from build123d import *

# Parameters (mm, degrees)
F1_DEPTH  = 8
F2_R      = 5.45
F3_DEPTH  = 1
F3_TAPER  = 20
F5_DEPTH  = 1
F5_TAPER  = 20
F6_R      = 2.15
F7_DEPTH  = 0.63
F8_W      = 90.39
F8_H      = 51.7
F9_DEPTH  = 1.5
F11_DEPTH = 0.58


with BuildPart() as f1:
    # F0 (on Front) → F1 (new body)
    with BuildSketch(Plane.XZ):
        with BuildLine():
            ThreePointArc((-61.915, -20.125), (-59.2320981157, -26.6020981157), (-52.755, -29.285))
            Line((-52.755, -29.285), (52.755, -29.285))
            ThreePointArc((52.755, -29.285), (59.2320981157, -26.6020981157), (61.915, -20.125))
            Line((61.915, -20.125), (61.915, 20.125))
            ThreePointArc((61.915, 20.125), (59.2320981157, 26.6020981157), (52.755, 29.285))
            Line((52.755, 29.285), (-52.755, 29.285))
            ThreePointArc((-52.755, 29.285), (-59.2320981157, 26.6020981157), (-61.915, 20.125))
            Line((-61.915, 20.125), (-61.915, -20.125))
        make_face()
    extrude(amount=-F1_DEPTH)

    # F2 (on face) → F3 (cut)
    with BuildSketch(Plane.XZ):
        with Locations((-52.765, 0)):
            Circle(F2_R)
    extrude(amount=-F3_DEPTH, taper=F3_TAPER, mode=Mode.SUBTRACT)

    # F4 (on face) → F5 (cut)
    with BuildSketch(Plane.XZ):
        with BuildLine():
            ThreePointArc((52.315, 5.4), (51.165, 6.55), (50.015, 5.4))
            Line((50.015, 5.4), (50.015, -5.4))
            ThreePointArc((50.015, -5.4), (51.165, -6.55), (52.315, -5.4))
            Line((52.315, -5.4), (52.315, 5.4))
        make_face()
    extrude(amount=-F5_DEPTH, taper=F5_TAPER, mode=Mode.SUBTRACT)

    # F6 (on face) → F7 (join)
    with BuildSketch(Plane.XY.offset(29.285)):
        with Locations((20.695, 4.44)):
            Circle(F6_R)
        with Locations((30.985, 4.44)):
            Circle(F6_R)
        with BuildLine():
            Line((43.905, 5.55), (40.205, 5.55))
            ThreePointArc((40.205, 5.55), (39.4978932188, 5.2571067812), (39.205, 4.55))
            Line((39.205, 4.55), (39.205, 4.35))
            ThreePointArc((39.205, 4.35), (39.4978932188, 3.6428932188), (40.205, 3.35))
            Line((40.205, 3.35), (43.905, 3.35))
            ThreePointArc((43.905, 3.35), (44.6121067812, 3.6428932188), (44.905, 4.35))
            Line((44.905, 4.35), (44.905, 4.55))
            ThreePointArc((44.905, 4.55), (44.6121067812, 5.2571067812), (43.905, 5.55))
        make_face()
    extrude(amount=F7_DEPTH)

    # F8 (on face) → F9 (cut)
    with BuildSketch(Plane.XZ):
        Rectangle(F8_W, F8_H)
    extrude(amount=-F9_DEPTH, mode=Mode.SUBTRACT)

    # F10 (on face) → F11 (join)
    with BuildSketch(Plane.YZ.offset(61.915)):
        with BuildLine():
            Line((4.54, -9.985), (4.34, -9.985))
            ThreePointArc((4.34, -9.985), (3.6328932188, -10.2778932188), (3.34, -10.985))
            Line((3.34, -10.985), (3.34, -18.485))
            ThreePointArc((3.34, -18.485), (3.6328932188, -19.1921067812), (4.34, -19.485))
            Line((4.34, -19.485), (4.54, -19.485))
            ThreePointArc((4.54, -19.485), (5.2471067812, -19.1921067812), (5.54, -18.485))
            Line((5.54, -18.485), (5.54, -10.985))
            ThreePointArc((5.54, -10.985), (5.2471067812, -10.2778932188), (4.54, -9.985))
        make_face()
    extrude(amount=F11_DEPTH)


solid = f1.part
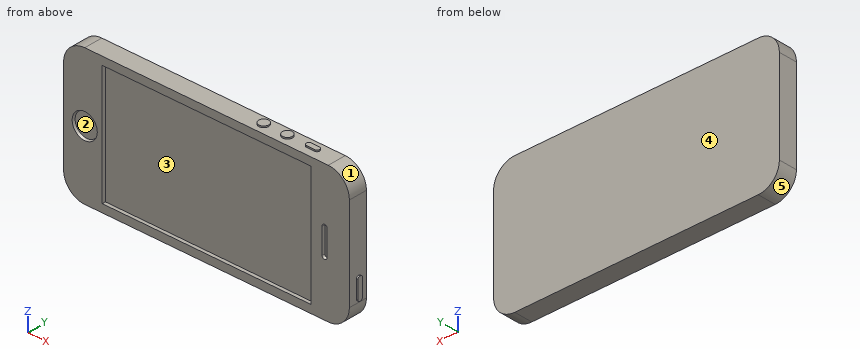
Geometry check sheet. Reference: the model listing, model coordinates, mm. Face numbers are marked on the shaded views. A direction names the side the tool comes from. Give positions to 0.01 mm unless a question says otherwise; leave off trailing zeros. Loops run counter-clockwise (first coordinate to the right, second up) from the corner with the lowest first, then second, coordinate; pieces in that order, holes last. Notation, with made-up numbers: M 45.25,36 L 73.25,36 A27 cw 73.25,56 Z; hole C 4.5,89.25 d11. An arc over 180 degrees is marked long. Write each question's results on one line, items separated by ' | '.
1) Thickness scan on line 1 (X direction, y = 0.75, z = -19) (3 decimals); line 2 (Z direction, x = 18.5, y = 0.5) (3 decimals); line 3 (X direction, y = 5.75, z = 3.5) (3 decimals). Record the ranges inside material, lowest first.
Answers follow:
line 1: -61.915 to -45.195, 45.195 to 61.915 | line 2: -29.285 to -25.85, 25.85 to 29.285 | line 3: -61.915 to 61.915
2) Tool access check on the marked faces 1 and 2. Record the directions out of +Z, -Z, +X, -X, +Y, -Y that give a thin tool (end or side, any length) a straight path to the whole face; none if there is none.
Answers follow:
face 1: +Z, +X, +Y, -Y | face 2: -Y
3) Release check for a two-part mould opening along X. For the marked faces 3, 4 and 5 record: +X half, -X half, draft (parallel to the pull), parting line (faces both ways), or undercut.
Answers follow:
face 3: undercut | face 4: draft | face 5: -X half
4) Section check B-B, the plane z = 14.5. Record the boundary of the cut face in (x, y) (3 decimals), plus the area to 3 significant figures.
Answers follow:
outline: M -61.915,0 L -45.195,0 L -45.195,1.5 L 45.195,1.5 L 45.195,0 L 61.915,0 L 61.915,8 L -61.915,8 Z | area: 855 mm2
5) Gauge pin test, flat ends, axial feed: pin 1 (2.5 mm diameter, centred on y = 3.5, z = -5.5, fed in from +X) (3 decimals); pin 2 (12 mm diameter, centred on x = 44, z = 22.5, fed in from -Y); pin 3 (2 mm diameter, centred on x = -13, z = -5.5, fed in from -Y); pin 4 (0.5 mm diameter, centred on x = 62.5, z = -16, fed in from +Y). Record the tip position at first contact, or that the pin passes through.
Answers follow:
pin 1: x = 61.915 | pin 2: y = 0 | pin 3: y = 1.5 | pin 4: y = 5.54
6) Section check A-A, the plane x = -43.5. Record the boundary of the cut face in (y, z) (3 decimals).
Answers follow:
outline: M 0,-29.285 L 8,-29.285 L 8,29.285 L 0,29.285 L 0,25.85 L 1.5,25.85 L 1.5,-25.85 L 0,-25.85 Z
